Solid Edge part; units mm, degrees
sketch "Sketch1" plane through (0, 0, 0) normal (0, 0, 1) x (1, 0, 0)
  line L0 (-30, -17.5) -> (30, -17.5)
  line L1 (30, -17.5) -> (30, 17.5)
  line L2 (30, 17.5) -> (-30, 17.5)
  line L3 (-30, 17.5) -> (-30, -17.5)
  circle A0 centre (-27.5, -15) radius 1.5
  circle A1 centre (-27.5, 15) radius 1.5
  circle A2 centre (27.5, -15) radius 1.5
  circle A3 centre (27.5, 15) radius 1.5
extrude "Protrusion1" add sketch "Sketch1" along normal blind 1.6
sketch "Sketch2" plane through (0, 0, 1.6) normal (0, 0, 1) x (1, 0, 0)
  line L0 (-39, 8.5) -> (-39, -8.5)
  line L1 (-39, -8.5) -> (-21, -8.5)
  line L2 (-21, -8.5) -> (-21, 8.5)
  line L3 (-21, 8.5) -> (-39, 8.5)
extrude "ExtrudedProtrusion_2" add sketch "Sketch2" along normal blind 5
sketch "Sketch3" plane through (0, 0, 1.6) normal (0, 0, 1) x (1, 0, 0)
  line L0 (-23.6555, 12.416) -> (-16.6555, 12.416)
  line L1 (-16.6555, 12.416) -> (-16.6555, 16.416)
  line L2 (-16.6555, 16.416) -> (-23.6555, 16.416)
  line L3 (-23.6555, 16.416) -> (-23.6555, 12.416)
  line L4 (27.8474, -13.0476) -> (27.8474, -7.0476)
  line L5 (27.8474, -7.0476) -> (22.8474, -7.0476)
  line L6 (22.8474, -7.0476) -> (22.8474, -13.0476)
  line L7 (22.8474, -13.0476) -> (27.8474, -13.0476)
extrude "ExtrudedProtrusion_3" add sketch "Sketch3" along normal blind 4
sketch "Sketch4" plane through (0, 0, 0) normal (0, 0, -1) x (1, 0, 0)
  line L0 (12, 6.9) -> (-2, 6.9)
  line L1 (-2, 6.9) -> (-2, -8.1)
  line L2 (-2, -8.1) -> (12, -8.1)
  line L3 (12, -8.1) -> (12, 6.9)
extrude "ExtrudedProtrusion_4" add sketch "Sketch4" along normal blind 4.3
properties material "Polycarbonate"
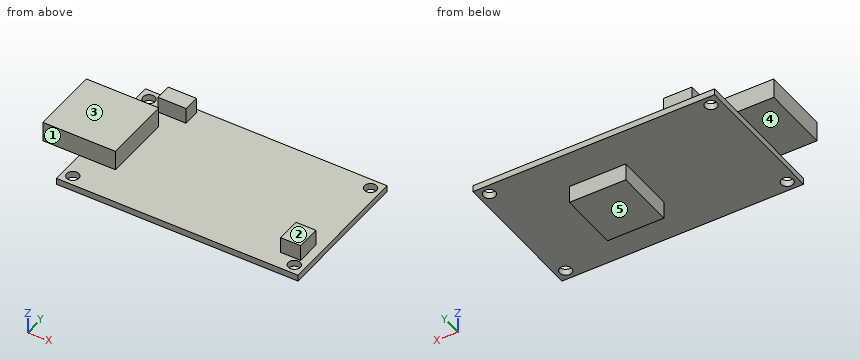
Input: part model. Units: mm. Frame: model coordinates. Face numbers are marked on the shaded views. A direction names the side the tool comes from. Round coordinates to 2 decimals unless told otherwise and drop trailing zeros. Order: outer loops, then holes, each group sorted by start corner. A loop starts at its lowest first (then second) coordinate and runs counter-clockwise, first axis right, second up. Notation, with made-up numbers: (17.25, 51) - (27.25, 51) arc R3 cw to (27.25, 55) - close; hole circle Ø8 at (-30.5, 66.5). An arc over 180 degrees is marked (long way). Use a Markdown table: item, result.
1. First-contact query: pin 1 (8 mm diameter, centred on x = -9.5, y = 3.5, fed in from -Z); pin 2 (2.5 mm diameter, centred on x = 25, y = -10, fed in from +Z); pin 3 (4 mm diameter, centred on y = -1, z = 5, fed in from +X); pin 4 (4.5 mm diameter, centred on y = -9, z = 4.5, fed in from -X). Flat tips, straight axial feed; report the tip coordinate or a pass-through.
Evaluation:
| item | result |
|---|---|
| pin 1 | z = 0 |
| pin 2 | z = 5.6 |
| pin 3 | x = -21 |
| pin 4 | x = -39 |
2. Section C-C on z = 0.75. Return the cut outline in (x, y).
Evaluation:
| item | result |
|---|---|
| outline | (-30, -17.5) - (30, -17.5) - (30, 17.5) - (-30, 17.5) - close; hole circle Ø3 at (-27.5, -15); hole circle Ø3 at (-27.5, 15); hole circle Ø3 at (27.5, -15); hole circle Ø3 at (27.5, 15) |
3. Section D-D on x = 24. Return the cut outline in (y, z).
Evaluation:
| item | result |
|---|---|
| outline | (-17.5, 0) - (17.5, 0) - (17.5, 1.6) - (-7.05, 1.6) - (-7.05, 5.6) - (-13.05, 5.6) - (-13.05, 1.6) - (-17.5, 1.6) - close |
4. Section A-A on y = -15. Return the cut outline in (x, z).
Evaluation:
| item | result |
|---|---|
| outline | (-30, 0) - (-29, 0) - (-29, 1.6) - (-30, 1.6) - close; (-26, 0) - (26, 0) - (26, 1.6) - (-26, 1.6) - close; (29, 0) - (30, 0) - (30, 1.6) - (29, 1.6) - close |
5. Access query for the marked faces 1, 2, 3, 4 and 5. Directions: +Z, -Z, +X, -X, +Y, -Y. A direction counts if a zero-diameter tool reaches every point of the face in a straight line with its end or side. Return the directions, or none.
Evaluation:
| item | result |
|---|---|
| face 1 | +Z, -X, -Y |
| face 2 | +Z, +X, +Y, -Y |
| face 3 | +Z, +X, -X, +Y, -Y |
| face 4 | -Z, -X, +Y, -Y |
| face 5 | -Z, +X, -X, +Y, -Y |
6. Material intervals for probe 1 along Y at (x, z) = (-27.5, 0.5); probe 2 along X at (y, z) = (-15.5, 1); probe 3 along Y at (x, z) = (-28, 0.5), sorted ascending.
Evaluation:
| item | result |
|---|---|
| probe 1 | -17.5 to -16.5, -13.5 to 13.5, 16.5 to 17.5 |
| probe 2 | -30 to -28.91, -26.09 to 26.09, 28.91 to 30 |
| probe 3 | -17.5 to -16.41, -13.59 to 13.59, 16.41 to 17.5 |
7. Section B-B on x = -27.5. Return the cut outline in (y, z).
Evaluation:
| item | result |
|---|---|
| outline | (-17.5, 0) - (-16.5, 0) - (-16.5, 1.6) - (-17.5, 1.6) - close; (-13.5, 0) - (13.5, 0) - (13.5, 1.6) - (8.5, 1.6) - (8.5, 6.6) - (-8.5, 6.6) - (-8.5, 1.6) - (-13.5, 1.6) - close; (16.5, 0) - (17.5, 0) - (17.5, 1.6) - (16.5, 1.6) - close |
